For this review, take the finished solid that the model builds, in its own axes (mm). A direction names the side the tool comes from. Coordinates: 2 decimals unless noted, no trailing zeros. Write each loop counter-clockwise with the first axis right and the second up, starting at its lowest first coordinate (ties: lowest second). Pieces come first, ordered by that corner, then holes. Notation, with made-up numbers: (-5.75, -17) -> (45.25, -17) arc R8 ccw to (45.25, -5) -> close; hole circle Ø7 at (20.25, 14.25). An arc over 180 degrees is marked (long way). One line per item, written item: value. Start each with the question number.
1) Add section A-A (x = 0). State the section outline as (y, z) points, and give its area (3 significant figures).
2) Add section B-B (z = 0). State the section outline as (x, y) points, and give its area (3 significant figures).
3) For probe 1 along Z at (x, y) = (-0.5, 34); probe 2 along X at (y, z) = (0.05, 0); probe 3 along Y at (x, z) = (-32, -11.5), list the stretches that pass through material, from the lowest coordinate up. Write a range as from..to.
4) Machinability: for faces 3 (the flat face through (-1, -1, -11)), 4 (the cylindrical face through (19.334, 20.227, -2.539)), which of the approach directions +Z, -Z, +X, -X, +Y, -Y give a long, thin tool a straight path to every point of the face, cutting with its end or side? Answer none if there is none.
5) Add section C-C (y = -10.5). State the section outline as (x, z) points, and give its area (3 significant figures).
6) Mouldability with a two-part tool opening along X and no side actions: class faces 1 (the flat face through (5, 40, -9)), 2 (the flat face through (20, 1, -1)) as released by +X, released by -X, zero draft, split by the parting line, or undercut.
7) For pin 1 Ø6 at (y, z) = (29, -29) entering from +X; pin 2 Ø5 at (x, z) = (-71.5, 72.5) entering from +Y; pin 3 Ø4 at (x, z) = (-40, -76) entering from +Y; pin 4 Ø18 at (x, z) = (0, 0) entering from -Y, all flat-tipped, find the tip position at first contact; note any pin that passes through.
from build123d import *

# Parameters (mm, degrees)
SKETCH1_R           = 40
SKETCH3_R           = 82.354581533
BOSS_EXTRUDE1_DEPTH = 1
SKETCH4_R           = 19.5
SKETCH4_R_2         = 10
BOSS_EXTRUDE2_DEPTH = 39
SKETCH5_R           = 10
CUT_EXTRUDE1_DEPTH  = 42.0000001


with BuildPart() as part:
    # Sketch1 → Revolve1 (revolve)
    with BuildSketch(Plane.XY):
        with Locations((87.5, 0)):
            Circle(SKETCH1_R)
    revolve(axis=Axis((0, -1000, 0), (0, 1, 0)))

    # Sketch3 → Boss-Extrude1 (add, symmetric)
    with BuildSketch(Plane(origin=(0, 0, 0), x_dir=(1, 0, 0), z_dir=(0, 1, 0))):
        Circle(SKETCH3_R)
    extrude(amount=BOSS_EXTRUDE1_DEPTH, both=True)

    # Sketch4 → Boss-Extrude2 (add)
    with BuildSketch(Plane(origin=(0, 1, 0), x_dir=(1, 0, 0), z_dir=(0, 1, 0))):
        with Locations(Location((0, 0, 0), (0, 0, 270))):  # turned: the seam where the file's is
            Circle(SKETCH4_R)
        with Locations(Location((0, 0, 0), (0, 0, 270))):  # turned: the seam where the file's is
            Circle(SKETCH4_R_2, mode=Mode.SUBTRACT)
    extrude(amount=BOSS_EXTRUDE2_DEPTH)

    # Sketch5 → Cut-Extrude1 (cut, through all)
    with BuildSketch(Plane(origin=(0, 1, 0), x_dir=(1, 0, 0), z_dir=(0, 1, 0))):
        with Locations(Location((0, 0, 0), (0, 0, 270))):  # turned: the seam where the file's is
            Circle(SKETCH5_R)
    extrude(amount=-CUT_EXTRUDE1_DEPTH, mode=Mode.SUBTRACT)


solid = part.part
Numbers:
1. outline: (-1, -47.51) arc R40 ccw (long way) to (1, -47.51) -> (1, -19.5) -> (40, -19.5) -> (40, -10) -> (-1, -10) -> close; (-1, 10) -> (40, 10) -> (40, 19.5) -> (1, 19.5) -> (1, 47.51) arc R40 ccw (long way) to (-1, 47.51) -> close
1. area: 10,900 mm²
2. outline: (-47.51, -1) -> (-10, -1) -> (-10, 40) -> (-19.5, 40) -> (-19.5, 1) -> (-47.51, 1) arc R40 ccw (long way) to start; (10, -1) -> (47.51, -1) arc R40 ccw (long way) to (47.51, 1) -> (19.5, 1) -> (19.5, 40) -> (10, 40) -> close
2. area: 10,900 mm²
3. probe 1: -108.57..-66.43, -19.49..-9.99, 9.99..19.49, 66.43..108.57
3. probe 2: -127.5..-10, 10..127.5
3. probe 3: -1..1
4. face 3: -Y
4. face 4: +Y
5. outline: circle Ø252.19 at (0, 0); hole circle Ø97.81 at (0, 0)
5. area: 42,400 mm²
6. face 1: zero draft
6. face 2: undercut
7. pin 1: x = 114.38
7. pin 2: y = 38.21
7. pin 3: y = 40
7. pin 4: through
